```python
from build123d import *

# Parameters (mm, degrees)
SKETCH1_W      = 79.70776103
SKETCH1_H      = 71.652189437
SKETCH1_W_2    = 59.70776103
SKETCH1_H_2    = 51.652189437
EXTRUDE1_DEPTH = 10
FILLET1_R      = 2


with BuildPart() as part:
    # Sketch1 → Extrude1 (new body)
    with BuildSketch(Plane(origin=(0, 0, 0), x_dir=(1, 0, 0), z_dir=(0, 1, 0))):
        with Locations((-2.013892898, -0.953949268)):
            Rectangle(SKETCH1_W, SKETCH1_H)
        with Locations((-2.013892898, -0.953949268)):
            Rectangle(SKETCH1_W_2, SKETCH1_H_2, mode=Mode.SUBTRACT)
    extrude(amount=EXTRUDE1_DEPTH)

    # Fillet1
    fillet1_edges = [part.edges().sort_by_distance(p)[0] for p in [
        (-41.867773413, 5, -34.872145451),
        (37.839987617, 5, -34.872145451),
        (-2.013892898, 0, -34.872145451),
        (-2.013892898, 10, -34.872145451),
        (37.839987617, 5, 36.780043986),
        (37.839987617, 0, 0.953949268),
        (37.839987617, 10, 0.953949268),
        (-41.867773413, 5, 36.780043986),
        (-2.013892898, 0, 36.780043986),
        (-2.013892898, 10, 36.780043986),
        (-41.867773413, 0, 0.953949268),
        (-41.867773413, 10, 0.953949268),
        (-31.867773413, 5, -24.872145451),
        (-31.867773413, 5, 26.780043986),
        (-31.867773413, 0, 0.953949268),
        (-31.867773413, 10, 0.953949268),
        (27.839987617, 5, 26.780043986),
        (-2.013892898, 0, 26.780043986),
        (-2.013892898, 10, 26.780043986),
        (27.839987617, 5, -24.872145451),
        (27.839987617, 0, 0.953949268),
        (27.839987617, 10, 0.953949268),
        (-2.013892898, 0, -24.872145451),
        (-2.013892898, 10, -24.872145451),
    ]]
    fillet(fillet1_edges, radius=FILLET1_R)


solid = part.part
```
CAD build for the part. Positions are in the model's coordinates, mm. A direction names the side the tool comes from. Round coordinates to 2 decimals unless told otherwise and drop trailing zeros. Order: outer loops, then holes, each group sorted by start corner. A loop starts at its lowest first (then second) coordinate and runs counter-clockwise, first axis right, second up.
Q1. Two-plate mould, pull along X, no slides. Class faces 6 (the cylindrical face through (28.41, 0.6, 0.62)), 7 (the cylindrical face through (37.27, 0.6, 0.48)), 8 (the flat face through (-3, 5, -34.872)): pulls with the +X half, pulls with the -X half, needs draft (parallel to the pull), parting line crosses it, or undercut.
Q2. Slice it at C-C (y = 4.5). Write the cut outline in (x, z).
Q3. Slice it at B-B (z = 20). Write the cut outline in (x, y).
Q4. Wall check: L1, parallel to Z at x = -6, y = 4; L2, parallel to X at y = 3.75, z = 23.5; L3, parallel to X at y = 1, z = -6.5. Give the ranges that are in metal, low to high.
Q5. Slice it at A-A (x = 10). Write the cut outline in (y, z).
Q6. Which spindle directions (+Z, -Z, +X, -X, +Y, -Y) get a long thin tool onto all of the face, cutting with end or side? Do faces 1 (the cylindrical face through (-41.297, 5.042, 36.179)), 2 (the cylindrical face through (-1.62, 0.6, 27.35)), 3 (the cylindrical face through (-32.44, 9.4, 0.62)), 4 (the cylindrical face through (-1.48, 9.4, 36.21)), 5 (the flat face through (-31.868, 5, 1)). Say none if no direction does.
Q7. Drop flat-ended pins along their axis: pin 1 (1 mm diameter, centred on y = 8.5, z = -9, fed in from -X); pin 2 (1.5 mm diameter, centred on x = -23.5, y = 9, fed in from -Z). Give the stop position or say it passes through.
Results below:
1. face 6: undercut
1. face 7: pulls with the +X half
1. face 8: needs draft
2. outline: (-41.87, -32.87) arc R2 ccw to (-39.87, -34.87) - (35.84, -34.87) arc R2 ccw to (37.84, -32.87) - (37.84, 34.78) arc R2 ccw to (35.84, 36.78) - (-39.87, 36.78) arc R2 ccw to (-41.87, 34.78) - close; hole (-31.87, -22.87) arc R2 ccw to (-29.87, -24.87) - (25.84, -24.87) arc R2 ccw to (27.84, -22.87) - (27.84, 24.78) arc R2 ccw to (25.84, 26.78) - (-29.87, 26.78) arc R2 ccw to (-31.87, 24.78) - close
3. outline: (-41.87, 2) arc R2 ccw to (-39.87, 0) - (-33.87, 0) arc R2 ccw to (-31.87, 2) - (-31.87, 8) arc R2 ccw to (-33.87, 10) - (-39.87, 10) arc R2 ccw to (-41.87, 8) - close; (27.84, 2) arc R2 ccw to (29.84, 0) - (35.84, 0) arc R2 ccw to (37.84, 2) - (37.84, 8) arc R2 ccw to (35.84, 10) - (29.84, 10) arc R2 ccw to (27.84, 8) - close
4. L1: z = -34.87 to -24.87, 26.78 to 36.78
4. L2: x = -41.87 to -31.87, 27.84 to 37.84
4. L3: x = -41.6 to -32.14, 28.11 to 37.57
5. outline: (0, -32.87) arc R2 ccw to (2, -34.87) - (8, -34.87) arc R2 ccw to (10, -32.87) - (10, -26.87) arc R2 ccw to (8, -24.87) - (2, -24.87) arc R2 ccw to (0, -26.87) - close; (0, 28.78) arc R2 ccw to (2, 26.78) - (8, 26.78) arc R2 ccw to (10, 28.78) - (10, 34.78) arc R2 ccw to (8, 36.78) - (2, 36.78) arc R2 ccw to (0, 34.78) - close
6. face 1: +Z, -X, +Y, -Y
6. face 2: -Y
6. face 3: +Y
6. face 4: +Z, +X, -X, +Y
6. face 5: +Y, -Y
7. pin 1: stops at x = -41.87
7. pin 2: stops at z = -34.86
